Build history of the part. All positions in model axes, mm. Face numbers are marked on the shaded views. Give positions to 0.01 mm unless a question says otherwise; leave off trailing zeros. Write each loop counter-clockwise with the first axis right and the second up, starting at its lowest first coordinate (ties: lowest second). Pieces come first, ordered by that corner, then holes. Notation, with made-up numbers: M 30.5,-33.5 L 56.5,-33.5 A29 ccw 56.5,2.5 Z; hole C 40,75 d10. An arc over 180 degrees is marked long. Return JSON: item names as keys, results as strings. Group by question number.
Q1. Band-saw the part on A-A, the plane z = 0. Give the cut face in (x, y) (3 decimals).
Q2. Band-saw the part on D-D, the plane y = -232. Give the cut face in (x, z), then the cut area to 3 significant figures.
Q3. Band-saw the part on C-C, the plane z = -76.2. Give the cut face in (x, y), then the cut area to 3 significant figures.
Q4. Band-saw the part on B-B, the plane x = -11. Give the cut face in (y, z) (3 decimals).
Q5. Wall check: probe 1 along X at (y, z) = (-157, 0); probe 2 along X at (y, z) = (-4, 38); probe 3 along Z at (x, y) = (38.1, -7.25). Give the ranges that are in metal, low to high.
Q6. Flat gauge pins, fed straight in: pin 1 Ø1.5 at (y, z) = (-247.5, -48) entering from +X; pin 2 Ø9.5 at (x, z) = (65.99, -38.1) entering from -Y; pin 3 Ø10 at (y, z) = (-240.5, -15) entering from -X; pin 4 Ø13.5 at (x, z) = (65.99, 38.1) entering from +Y. Where does each tip first touch, or does it go through?
Q7. Pull direction X, two halves, no side cores. Call the marked faces 1, 2 and 3: +X half, -X half, draft (parallel to the pull), parting line (faces both ways), or undercut.
from build123d import *

# Parameters (mm, degrees)
F_5_16_CLEARANCE_HOLE1_D = 8.4328
CIRPATTERN1_COUNT        = 12


with BuildPart() as part:
    # Sketch1 → Revolve1 (revolve)
    with BuildSketch(Plane.XY):
        Polygon((-57.15, 0), (-88.9, 0), (-88.9, -12.7), (-57.15, -12.7), (-57.15, -295.275), (-51.1302, -295.275), (-51.1302, -3.175), (-57.15, -3.175), align=None)
    revolve(axis=Axis((0, 0, 0), (0, -1, 0)))

    # 5/16 Clearance Hole1 (through all)
    with Locations(Plane(origin=(0, 0, 0), x_dir=(1, 0, 0), z_dir=(0, 1, 0))):
        with Locations((-76.2, 0)):
            f_5_16_clearance_hole1 = Hole(F_5_16_CLEARANCE_HOLE1_D / 2)

    # CirPattern1: 5/16 Clearance Hole1 ×12 about axis
    cirpattern1_axis = Axis((0, 0, 0), (0, 1, 0))
    for i in range(1, CIRPATTERN1_COUNT):
        add(f_5_16_clearance_hole1.rotate(cirpattern1_axis, i * 360 / CIRPATTERN1_COUNT), mode=Mode.SUBTRACT)


solid = part.part
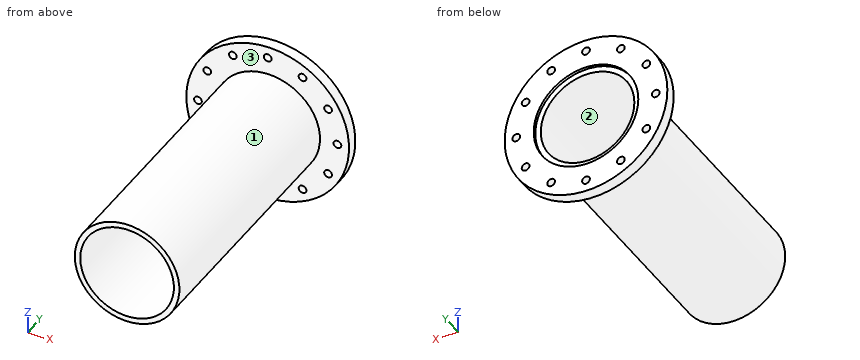
From the geometry:
{
 "1": {"outline": "M -88.9,-12.7 L -80.416,-12.7 L -80.416,0 L -88.9,0 Z; M -71.984,-12.7 L -57.15,-12.7 L -57.15,-295.275 L -51.13,-295.275 L -51.13,-3.175 L -57.15,-3.175 L -57.15,0 L -71.984,0 Z; M 51.13,-295.275 L 57.15,-295.275 L 57.15,-12.7 L 71.984,-12.7 L 71.984,0 L 57.15,0 L 57.15,-3.175 L 51.13,-3.175 Z; M 80.416,-12.7 L 88.9,-12.7 L 88.9,0 L 80.416,0 Z"},
 "2": {"outline": "C 0,0 d114.3; hole C 0,0 d102.26", "area": "2,050 mm^2"},
 "3": {"outline": "M -45.79,-12.7 L -4.22,-12.7 L -4.22,0 L -45.79,0 Z; M 4.22,-12.7 L 45.79,-12.7 L 45.79,0 L 4.22,0 Z", "area": "1,060 mm^2"},
 "4": {"outline": "M -295.275,-56.081 L -12.7,-56.081 L -12.7,-88.217 L 0,-88.217 L 0,-56.081 L -3.175,-56.081 L -3.175,-49.933 L -295.275,-49.933 Z; M -295.275,49.933 L -3.175,49.933 L -3.175,56.081 L 0,56.081 L 0,88.217 L -12.7,88.217 L -12.7,56.081 L -295.275,56.081 Z"},
 "5": {"probe 1": "x = -57.15 to -51.13, 51.13 to 57.15", "probe 2": "x = -80.37 to -70.21, -61.78 to -34.21, 34.21 to 61.78, 70.21 to 80.37", "probe 3": "z = -80.32 to -70.21, -61.77 to -34.1, 34.1 to 61.77, 70.21 to 80.32"},
 "6": {"pin 1": "stops at x = 32.15", "pin 2": "stops at y = -12.7", "pin 3": "stops at x = -56.27", "pin 4": "stops at y = 0"},
 "7": {"face 1": "parting line", "face 2": "undercut", "face 3": "draft"}
}
